from build123d import *

# Parameters (mm, degrees)
SKETCH1_R           = 45
BOSS_EXTRUDE1_DEPTH = 3
CUT_EXTRUDE1_DEPTH  = 3
SKETCH4_R           = 1.5
CUT_EXTRUDE2_DEPTH  = 3


with BuildPart() as part:
    # Sketch1 → Boss-Extrude1 (new body)
    with BuildSketch(Plane(origin=(0, 0, 0), x_dir=(1, 0, 0), z_dir=(0, 1, 0))):
        with Locations(Location((0, 0, 0), (0, 0, 270))):
            Circle(SKETCH1_R)
    extrude(amount=BOSS_EXTRUDE1_DEPTH)

    # Sketch3 → Cut-Extrude1 (cut)
    with BuildSketch(Plane(origin=(0, 3, 0), x_dir=(1, 0, 0), z_dir=(0, 1, 0))):
        with BuildLine():
            Line((-25.882250574, 3.5), (0, 6.5))
            Line((0, 6.5), (25.882250574, 3.5))
            ThreePointArc((25.882250574, 3.5), (29, 0), (25.882250574, -3.5))
            Line((25.882250574, -3.5), (0, -6.5))
            Line((0, -6.5), (-25.882250574, -3.5))
            ThreePointArc((-25.882250574, -3.5), (-29, 0), (-25.882250574, 3.5))
        make_face()
    extrude(amount=-CUT_EXTRUDE1_DEPTH, mode=Mode.SUBTRACT)

    # Sketch4 → Cut-Extrude2 (cut)
    with BuildSketch(Plane(origin=(0, 3, 0), x_dir=(1, 0, 0), z_dir=(0, 1, 0))):
        with Locations(Location((-7, -10.5, 0), (0, 0, 270))):
            Circle(SKETCH4_R)
        with Locations(Location((7, -10.5, 0), (0, 0, 270))):
            Circle(SKETCH4_R)
        with Locations(Location((-7, 10.5, 0), (0, 0, 270))):
            Circle(SKETCH4_R)
        with Locations(Location((7, 10.5, 0), (0, 0, 270))):
            Circle(SKETCH4_R)
    extrude(amount=-CUT_EXTRUDE2_DEPTH, mode=Mode.SUBTRACT)


solid = part.part
Model file for the job. Use its own axes, mm. A direction names the side the tool comes from. Coordinates: 2 decimals unless noted, no trailing zeros. Write each loop counter-clockwise with the first axis right and the second up, starting at its lowest first coordinate (ties: lowest second). Pieces come first, ordered by that corner, then holes. Notation, with made-up numbers: (86.25, -10.5) -> (128.25, -10.5) arc R31 ccw to (128.25, 23.5) -> close; hole circle Ø3 at (30, -23). An arc over 180 degrees is marked (long way). One line per item, written item: value. Start each with the question number.
1) Slice it at A-A on z = 0. Write the cut outline in (x, y), then the cut area to 3 significant figures.
2) Slice it at C-C on y = 1.1. Write the cut outline in (x, z), then the cut area to 3 significant figures.
3) Slice it at D-D on x = -7. Write the cut outline in (y, z), then the cut area to 3 significant figures.
4) Which spindle directions (+Z, -Z, +X, -X, +Y, -Y) get a long thin tool onto all of the face, cutting with end or side? Do faces 4 (the face through (-29, 2, 0)), 5 (the face through (1, 3, 9)). Say none if no direction does.
5) Pull direction X, two halves, no side cores. Call faces 1 (the face through (13.12, 1.52, 4.98)), 2 (the face through (1, 0, 9)), 3 (the face through (-17.235, 1.479, 41.569)): +X half, -X half, draft (parallel to the pull), parting line (faces both ways), or undercut.
6) Probe probe 1 along X at (y, z) = (2, 10.5); probe 2 along Z at (x, y) = (-12.5, 1.65); probe 3 along X at (y, z) = (1.75, -0.5). List the from-to ranges inside material, lowest first.
7) Slice it at B-B on x = -20.5. Write the cut outline in (y, z), then the cut area to 3 significant figures.
Answers follow:
1. outline: (-45, 0) -> (-29, 0) -> (-29, 3) -> (-45, 3) -> close; (29, 0) -> (45, 0) -> (45, 3) -> (29, 3) -> close
1. area: 96.0 mm2
2. outline: circle Ø90 at (0, 0); hole (-25.88, -3.5) -> (0, -6.5) -> (25.88, -3.5) arc R3.52 ccw to (25.88, 3.5) -> (0, 6.5) -> (-25.88, 3.5) arc R3.52 ccw to start; hole circle Ø3 at (-7, -10.5); hole circle Ø3 at (-7, 10.5); hole circle Ø3 at (7, -10.5); hole circle Ø3 at (7, 10.5)
2. area: 5,780 mm2
3. outline: (0, -44.45) -> (3, -44.45) -> (3, -12) -> (0, -12) -> close; (0, -9) -> (3, -9) -> (3, -5.69) -> (0, -5.69) -> close; (0, 5.69) -> (3, 5.69) -> (3, 9) -> (0, 9) -> close; (0, 12) -> (3, 12) -> (3, 44.45) -> (0, 44.45) -> close
3. area: 215 mm2
4. face 4: +Y, -Y
4. face 5: +Z, -Z, +X, -X, +Y
5. face 1: undercut
5. face 2: draft
5. face 3: parting line
6. probe 1: -43.76 to -8.5, -5.5 to 5.5, 8.5 to 43.76
6. probe 2: -43.23 to -5.05, 5.05 to 43.23
6. probe 3: -45 to -28.96, 28.96 to 45
7. outline: (0, -40.06) -> (3, -40.06) -> (3, -4.12) -> (0, -4.12) -> close; (0, 4.12) -> (3, 4.12) -> (3, 40.06) -> (0, 40.06) -> close
7. area: 216 mm2
